Here's how the part is built. I have some questions about the finished solid (model axes, mm). A direction names the side the tool comes from. Coordinates: 2 decimals unless noted, no trailing zeros. Order: outer loops, then holes, each group sorted by start corner. A loop starts at its lowest first (then second) coordinate and runs counter-clockwise, first axis right, second up. Notation, with made-up numbers: (-0.5, -25) - (3.5, -25) arc R17 ccw to (3.5, -14) - close; hole circle Ø4 at (87.5, 40). An arc over 180 degrees is marked (long way). Use one line per item in the form item = value. Start each with the question number.
from build123d import *

# Parameters (mm, degrees)
SKETCH_1_W                     = 50
SKETCH_1_H                     = 50
EXTRUDE_1_DEPTH                = 8
HOLE_WIZARD_M22_1_D            = 26
HOLE_WIZARD_M3_5_1_D           = 4
HOLE_WIZARD_M3_5_1_CBORE_D     = 7
HOLE_WIZARD_M3_5_1_CBORE_DEPTH = 4
HOLE_WIZARD_4_2_4_2_1_D        = 4.2
HOLE_WIZARD_4_2_4_2_1_DEPTH    = 12.4
HOLE_WIZARD_4_2_4_2_1_TIP      = 1.2618073
FILLET_1_R                     = 15


with BuildPart() as part:
    # 草图1 → 凸台-拉伸1 (new body)
    with BuildSketch(Plane.XY.offset(8)):
        with Locations((39.062572137, 28.826485826)):
            Rectangle(SKETCH_1_W, SKETCH_1_H)
    extrude(amount=-EXTRUDE_1_DEPTH)

    # M22 间隙孔1 (through all)
    with Locations(Plane(origin=(0, 0, 0), x_dir=(-1, 0, 0), z_dir=(0, 0, -1))):
        with Locations((-39.062572137, 30.829359323)):
            Hole(HOLE_WIZARD_M22_1_D / 2)

    # M3.5 六角头机械螺钉的柱形沉头孔1 (through all)
    with Locations(Plane.XY.offset(8)):
        with Locations((39.062572137, 13.329359323), (39.062572137, 48.329359323), (56.562572137, 30.829359323), (21.562572137, 30.829359323)):
            CounterBoreHole(HOLE_WIZARD_M3_5_1_D / 2, HOLE_WIZARD_M3_5_1_CBORE_D / 2, HOLE_WIZARD_M3_5_1_CBORE_DEPTH)

    # Ø4.2 (4.2) 直径孔1
    with Locations(Plane(origin=(0, 3.826485826, 0), x_dir=(-1, 0, 0), z_dir=(0, -1, 0))):
        with Locations((-24.062572137, -4), (-54.062572137, -4)):
            Hole(HOLE_WIZARD_4_2_4_2_1_D / 2, depth=HOLE_WIZARD_4_2_4_2_1_DEPTH)
            with Locations((0, 0, -(HOLE_WIZARD_4_2_4_2_1_DEPTH + HOLE_WIZARD_4_2_4_2_1_TIP / 2))):  # 118° drill point
                Cone(0, HOLE_WIZARD_4_2_4_2_1_D / 2, HOLE_WIZARD_4_2_4_2_1_TIP, mode=Mode.SUBTRACT)

    # 圆角1
    fillet_1_edges = [part.edges().sort_by_distance(p)[0] for p in [
        (64.062572137, 53.826485826, 4),
        (14.062572137, 53.826485826, 4),
    ]]
    fillet(fillet_1_edges, radius=FILLET_1_R)


solid = part.part
1) Suppose I cut it at B-B, the plane y = 18.5. List the corners of the cut face in (x, z) for me, then the cut area to 3 significant figures.
2) Suppose I cut it at D-D, the plane y = 7.5. List the corners of the cut face in (x, z) for me.
3) For pin 1 (4 mm diameter, centred on x = 54.06, z = 4, fed in from -Y) (3 decimals); pin 2 (5 mm diameter, centred on x = 39.06, y = 48.33, fed in from -Z); pin 3 (3.5 mm diameter, centred on x = 39.06, y = 13.33, fed in from +Z); pin 4 (4 mm diameter, centred on x = 24.06, z = 4, fed in from +Y), each with a flat end and sliding along its axis, tell me the tip position at first contact or that it passes through.
4) Suppose I cut it at C-C, the plane z = 1. List the corners of the cut face in (x, y) for me.
5) Which directions (+Z, -Z, +X, -X, +Y, -Y) give clear straight access to the entire face, cutting with the end or side of a thin tool? Please do faces 1 (the conical face through (23.87, 17.27, 3.69)), 2 (the cylindrical face through (24.9, 31.88, 6.03)).
6) If we mould it in two halves opening along X, with no side actions, what happens to faces 3 (the cylindrical face through (59.6, 49.5, 3.9)), 4 (the flat face through (39, 53.826, 4)), 5 (the flat face through (23, 29, 4))? For each: pulls with the +X half, pulls with the -X half, needs draft (parallel to the pull), parting line crosses it, or undercut.
7) Suppose I cut it at A-A, the plane x = 27. List the corners of the cut face in (y, z) for me, then the cut area to 3 significant figures.
8) I need wall thicknesses on probe 1 along X at (y, z) = (31, 5); probe 2 along X at (y, z) = (28.5, 7); probe 3 along X at (y, z) = (42.5, 7). Which ranges of each line are inside material? Lowest first, please. Write a range as [from, to].
From the geometry:
q1.outline = (14.06, 0) - (34.94, 0) - (34.94, 8) - (14.06, 8) - close; (43.18, 0) - (64.06, 0) - (64.06, 8) - (43.18, 8) - close
q1.area = 334 mm2
q2.outline = (14.06, 0) - (64.06, 0) - (64.06, 8) - (14.06, 8) - close; hole circle Ø4.2 at (24.06, 4); hole circle Ø4.2 at (54.06, 4)
q3.pin_1 = 16.285
q3.pin_2 = 0
q3.pin_3 = through
q3.pin_4 = 53.52
q4.outline = (14.06, 3.83) - (64.06, 3.83) - (64.06, 38.83) arc R15 ccw to (49.06, 53.83) - (29.06, 53.83) arc R15 ccw to (14.06, 38.83) - close; hole circle Ø4 at (21.56, 30.83); hole circle Ø26 at (39.06, 30.83); hole circle Ø4 at (39.06, 13.33); hole circle Ø4 at (39.06, 48.33); hole circle Ø4 at (56.56, 30.83)
q5.face_1 = -Y
q5.face_2 = +Z
q6.face_3 = pulls with the +X half
q6.face_4 = needs draft
q6.face_5 = undercut
q7.outline = (3.83, 0) - (25.98, 0) - (25.98, 8) - (3.83, 8) - close; (35.68, 0) - (53.68, 0) - (53.68, 8) - (35.68, 8) - close
q7.area = 321 mm2
q8.probe_1 = [14.06, 18.07], [25.06, 26.06], [52.06, 53.07], [60.06, 64.06]
q8.probe_2 = [14.06, 18.95], [24.17, 26.27], [51.85, 53.95], [59.17, 64.06]
q8.probe_3 = [14.52, 33.34], [44.79, 63.61]
